Part model, mm, in its own coordinate system. A direction names the side the tool comes from. Give positions to 0.01 mm unless a question says otherwise; leave off trailing zeros. Write each loop counter-clockwise with the first axis right and the second up, starting at its lowest first coordinate (ties: lowest second). Pieces come first, ordered by that corner, then holes. Notation, with made-up numbers: M 86.25,-24 L 117.25,-24 A37 ccw 117.25,14 Z; hole C -0.75,-4 d8. An arc over 180 degrees is marked long. Answer as CSV lines item,"result". Start each with the question number.
1) Tool access for faces 1 (the cylindrical face through (28.9, -34.3, 3)), 2 (the cylindrical face through (31.86, 10.03, -9.86)): list every direction of +Z, -Z, +X, -X, +Y, -Y with a clear straight run to the whole face (end or side of a thin tool).
2) Slice it at A-A, the plane y = 0. Give the cut face in (x, z).
3) Slice it at C-C, the plane z = -6.25. Give the cut face in (x, y), plus the area to 3 significant figures.
4) Wall check: line 1 along Y through (x, z) = (0, -12.5); line 2 along Z through (x, y) = (-24, 34.5); line 3 along X through (y, z) = (-20.5, -18). Give the ranges that are in metal, low to high. Write a range as from..to.
5) Mould opens along Y. For faces 3 (the flat face through (38.1, 0, 3)), 4 (the cylindrical face through (-34.454, 29.227, 2.958)), 5 (the flat face through (0, -38.1, 3)) say: pulls with the +Y half, pulls with the -Y half, needs draft (parallel to the pull), parting line crosses it, or undercut.
6) Pin check, flat tips, straight feed: pin 1 Ø9 at (x, y) = (-30.76, 30.76) entering from -Z; pin 2 Ø10 at (y, z) = (11.5, -9) entering from +X. Stop position of each tip, or through.
Autodesk Inventor part; units mm, degrees
ref_plane "YZ Plane" through (0, 0, 0) normal (1, 0, 0) x (0, 1, 0)
ref_plane "XZ Plane" through (0, 0, 0) normal (0, 1, 0) x (-1, 0, 0)
ref_plane "XY Plane" through (0, 0, 0) normal (0, 0, 1) x (1, 0, 0)
sketch "Boceto1" plane through (0, 0, 0) normal (0, 0, 1) x (1, 0, 0)
  line L0 (38.1, -38.1) -> (-38.1, -38.1)
  line L1 (-38.1, -38.1) -> (-38.1, 38.1)
  line L2 (-38.1, 38.1) -> (38.1, 38.1)
  line L3 (38.1, 38.1) -> (38.1, -38.1)
  line L4 (38.1, -38.1) -> (-38.1, 38.1) construction
  line L5 (-38.1, -38.1) -> (38.1, 38.1) construction
  circle A0 centre (0, 0) radius 25.4
  circle A1 centre (0, 0) radius 33.4
  dimension "d0" = 76.2
  dimension "d1" = 76.2
  dimension "d2" = 50.8
  dimension "d3" = 8
extrude "Extrusión1" add sketch "Boceto1" along normal blind 6 contours L0 L1 L2 L3 | A1
extrude "Extrusión2" add sketch "Boceto1" against normal blind 20 contours A1
sketch "Boceto2" plane through (0, 0, 0) normal (0, 0, -1) x (-1, 0, 0)
  line L0 (-38.1, 38.1) -> (38.1, 38.1)
  circle A0 centre (0, 0) radius 25.4
  line L1 (38.1, 38.1) -> (38.1, -38.1)
  line L2 (38.1, -38.1) -> (-38.1, -38.1)
  line L3 (-38.1, -38.1) -> (-38.1, 38.1)
  circle A1 centre (30.7591, 30.7591) radius 4
  circle A2 centre (-30.7591, 30.7591) radius 4
  circle A3 centre (-30.7591, -30.7591) radius 4
  circle A4 centre (30.7591, -30.7591) radius 4
  dimension "d10" = 8
  dimension "d11" = 8
  dimension "d12" = 8
  dimension "d13" = 8
extrude "Extrusión3" cut sketch "Boceto2" against normal blind 20 contours A1 | A2 | A3 | A4
fillet "Empalme1" radius 3 4 edges at (-38.1, 38.1, 3) (38.1, 38.1, 3) (38.1, -38.1, 3) (-38.1, -38.1, 3)
properties part number "chumacera"
Found:
1,face 1,"+Z, -Z"
1,face 2,"-Z"
2,outline,"M -38.1,0 L -33.4,0 L -33.4,-20 L -25.4,-20 L -25.4,6 L -38.1,6 Z; M 25.4,-20 L 33.4,-20 L 33.4,0 L 38.1,0 L 38.1,6 L 25.4,6 Z"
3,outline,"C 0,0 d66.8; hole C 0,0 d50.8"
3,area,"1,480 mm²"
4,line 1,"-33.4..-25.4, 25.4..33.4"
4,line 2,"0..6"
4,line 3,"-26.37..-15, 15..26.37"
5,face 3,"needs draft"
5,face 4,"undercut"
5,face 5,"pulls with the -Y half"
6,pin 1,"z = 0"
6,pin 2,"x = 32.76"
